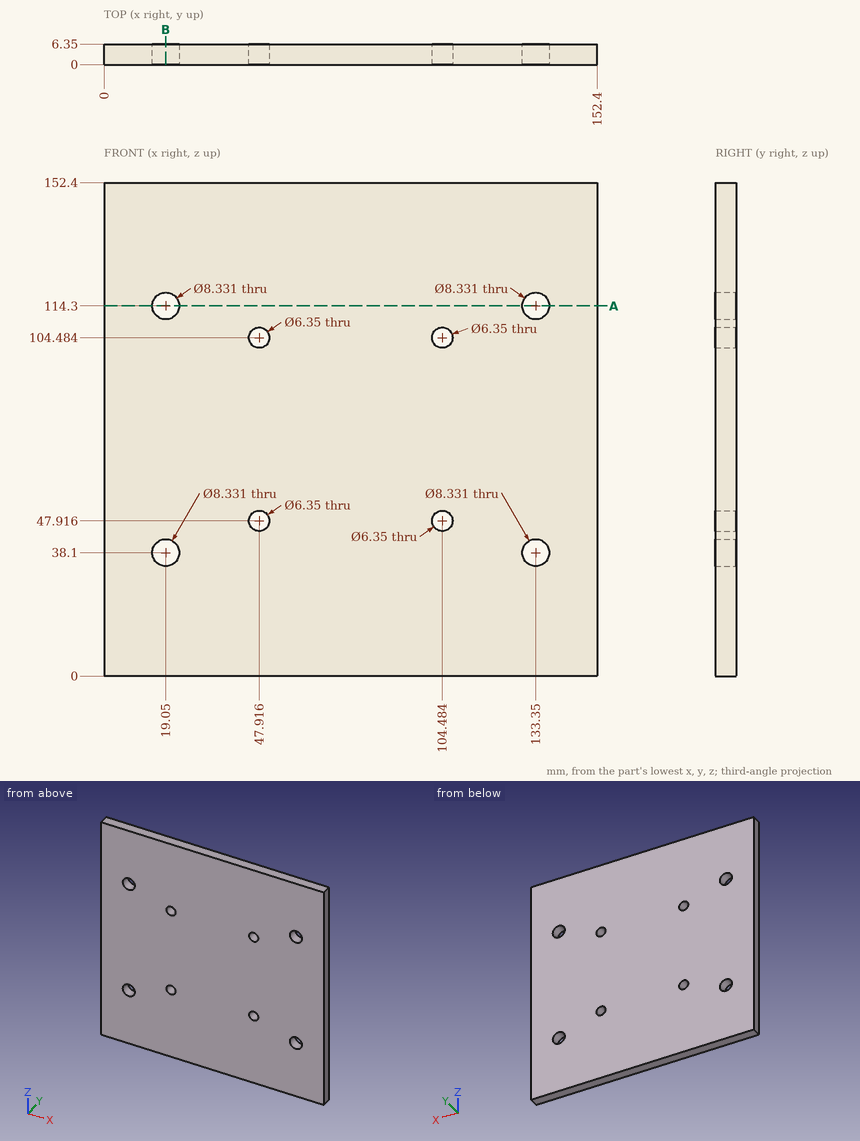
Here's the drawing with two shaded views (mm, measured from the low corner). I have some questions. Round coordinates to 2 decimals unless told otherwise and drop trailing zeros. Write each loop counter-clockwise with the first axis right and the second up, starting at its lowest first coordinate (ties: lowest second). Pieces come first, ordered by that corner, then holes. Notation, with made-up numbers: M 68.5,10.25 L 93.5,10.25 A20 cw 93.5,43.25 Z; hole C 11.25,45 d5. An arc over 180 degrees is marked long. Use CSV: the item, a comma, the result in double quotes.
(1) Imagine slicing it at B-B (x = 19.05). Write out the boundary of the cut face in (y, z), plus the area to 3 significant figures.
Check values:
outline,"M 0,0 L 6.35,0 L 6.35,33.93 L 0,33.93 Z; M 0,42.27 L 6.35,42.27 L 6.35,110.13 L 0,110.13 Z; M 0,118.47 L 6.35,118.47 L 6.35,152.4 L 0,152.4 Z"
area,"862 mm^2"
(2) I need wall thicknesses on line 1 along Z through (x, y) = (19.05, 2); line 2 along X through (y, z) = (3.25, 38.5); line 3 along X through (y, z) = (2, 102.5) (1 decimal). Which ranges of each line are inside material? Lowest first, please.
Check values:
line 1,"0 to 33.93, 42.27 to 110.13, 118.47 to 152.4"
line 2,"0 to 14.9, 23.2 to 129.2, 137.5 to 152.4"
line 3,"0 to 45.4, 50.4 to 102, 107 to 152.4"
(3) Imagine slicing it at A-A (z = 114.3). Write out the boundary of the cut face in (x, y).
Check values:
outline,"M 0,0 L 14.88,0 L 14.88,6.35 L 0,6.35 Z; M 23.22,0 L 129.18,0 L 129.18,6.35 L 23.22,6.35 Z; M 137.52,0 L 152.4,0 L 152.4,6.35 L 137.52,6.35 Z"
